from build123d import *

# Parameters (mm, degrees)
SKETCH1_R                    = 33.274
BOSS_EXTRUDE1_DEPTH          = 6.35
PLATEMTGSCREW_D              = 2.8702
PLATEMTGSCREW_DEPTH          = 10.1854
PLATEMTGSCREW_CSINK_D        = 7.7978
PLATEMTGSCREW_CSINK_ANGLE    = 82
PLATEMTGSCREW_TIP            = 0.862295074
ENCODERMTGHOLES_D            = 2.2606
SLIPRGSHFTCLR_D              = 13.09624
SLIPRGSHFTCLR_DEPTH          = 6.35
SLIPRGSHFTCLR_TIP            = 3.934507437
ADDITIONAL_HOLES_D           = 4.0386
ADDITIONAL_HOLES_CSINK_D     = 7.7978
ADDITIONAL_HOLES_CSINK_ANGLE = 82
CUT_EXTRUDE1_DEPTH           = 7.3500001


with BuildPart() as part:
    # Sketch1 → Boss-Extrude1 (new body)
    with BuildSketch(Plane(origin=(0, 0, 0), x_dir=(1, 0, 0), z_dir=(0, 1, 0))):
        Circle(SKETCH1_R)
    extrude(amount=BOSS_EXTRUDE1_DEPTH)

    # PlateMtgScrew
    with Locations(Plane(origin=(0, 6.35, 0), x_dir=(1, 0, 0), z_dir=(0, 1, 0))):
        with Locations((30.226, 0), (-30.226, 0), (0, -30.226)):
            CounterSinkHole(PLATEMTGSCREW_D / 2, PLATEMTGSCREW_CSINK_D / 2, depth=PLATEMTGSCREW_DEPTH, counter_sink_angle=PLATEMTGSCREW_CSINK_ANGLE)
            with Locations((0, 0, -(PLATEMTGSCREW_DEPTH + PLATEMTGSCREW_TIP / 2))):  # 118° drill point
                Cone(0, PLATEMTGSCREW_D / 2, PLATEMTGSCREW_TIP, mode=Mode.SUBTRACT)

    # EncoderMtgHoles (through all)
    with Locations(Plane(origin=(0, 6.35, 0), x_dir=(1, 0, 0), z_dir=(0, 1, 0))):
        with Locations((23.0124, 0), (-23.0124, 0)):
            Hole(ENCODERMTGHOLES_D / 2)

    # SlipRgShftClr
    with Locations(Plane(origin=(0, 6.35, 0), x_dir=(1, 0, 0), z_dir=(0, 1, 0))):
        with Locations((0, 0)):
            Hole(SLIPRGSHFTCLR_D / 2, depth=SLIPRGSHFTCLR_DEPTH)
            with Locations((0, 0, -(SLIPRGSHFTCLR_DEPTH + SLIPRGSHFTCLR_TIP / 2))):  # 118° drill point
                Cone(0, SLIPRGSHFTCLR_D / 2, SLIPRGSHFTCLR_TIP, mode=Mode.SUBTRACT)

    # Additional Holes (through all)
    with Locations(Plane(origin=(0, 6.35, 0), x_dir=(1, 0, 0), z_dir=(0, 1, 0))):
        with Locations((-9.898670365, 5.715), (9.898670365, 5.715)):
            CounterSinkHole(ADDITIONAL_HOLES_D / 2, ADDITIONAL_HOLES_CSINK_D / 2, counter_sink_angle=ADDITIONAL_HOLES_CSINK_ANGLE)

    # Sketch16 → Cut-Extrude1 (cut, through all)
    with BuildSketch(Plane(origin=(0, 6.35, 0), x_dir=(1, 0, 0), z_dir=(0, 1, 0))):
        Polygon((-192.02067324, 25.4), (-21.494163766, 25.4), (21.494163766, 25.4), (192.02067324, 25.4), (192.02067324, 366.453018948), (-192.02067324, 366.453018948), align=None)
    extrude(amount=-CUT_EXTRUDE1_DEPTH, mode=Mode.SUBTRACT)


solid = part.part
Design review of the part built by this model. Coordinates are the model's own, in mm. Give positions to 0.01 mm unless a question says otherwise; leave off trailing zeros. Loops run counter-clockwise (first coordinate to the right, second up) from the corner with the lowest first, then second, coordinate; pieces in that order, holes last. Notation, with made-up numbers: M 62.5,78.5 L 107.5,78.5 A16 cw 107.5,92.5 Z; hole C 3.5,15.25 d2. An arc over 180 degrees is marked long. One line per question, with ' | ' between items. Start each with the question number.
1. Add section A-A (z = 0). Write out the cut boundary in (x, y), plus the area to 3 significant figures.
2. To check wall thickness, follow L1, parallel to Z at x = 0, y = 3; L2, parallel to Z at x = -2, y = 5.75; L3, parallel to X at y = 2.75, z = -7. State the ranges of each line that lie inside material, in increasing order.
3. Insertion check: P1, Ø1.7, axis at x = 0, z = 30.226, coming from the +Y side; P2, Ø3, axis at x = 20, y = 5, coming from the +Z side; P3, Ø4.5, axis at x = -30.226, z = 0, coming from the +Y side. Each pin has a flat end and moves straight along its axis. Give the tip position at first contact, or say it passes through.
4. Add section C-C (y = 1.5). Give the number of separate pieces and of enclosed holes in the cut face, plus the area to 3 significant figures.
5. Add section B-B (x = 0). Write out the cut boundary in (y, z), plus the area to 3 significant figures.
6. Add section D-D (z = 24). Write out the cut boundary in (x, y), plus the area to 3 significant figures.
7. The part is to be moulded in two halves that separate along X. For faces 1 (the face through (-1.136, 3.131, 33.255)), 2 (the face through (0.311, 1.733, 31.627)), 3 (the face through (7, 6.35, 3)), 4 (the face through (0.202, 3.653, 28.684)), say which applies: released by +X, released by -X, zero draft, split by the parting line, or undercut.
Worked out:
1) outline: M -33.27,0 L -31.66,0 L -31.66,3.52 L -33.27,5.37 Z; M -28.79,0 L -24.14,0 L -24.14,6.35 L -26.33,6.35 L -28.79,3.52 Z; M -21.88,0 L -6.55,0 L -6.55,6.35 L -21.88,6.35 Z; M 6.55,0 L 21.88,0 L 21.88,6.35 L 6.55,6.35 Z; M 24.14,0 L 28.79,0 L 28.79,3.52 L 26.33,6.35 L 24.14,6.35 Z; M 31.66,0 L 33.27,0 L 33.27,5.37 L 31.66,3.52 Z | area: 261 mm²
2) L1: z = -25.4 to -6.55, 6.55 to 28.79, 31.66 to 33.27 | L2: z = -25.4 to -6.24, 6.24 to 27.5, 32.95 to 33.21 | L3: x = -32.53 to -11.46, -8.34 to 8.34, 11.46 to 32.53
3) P1: passes through | P2: stops at z = 27.66 | P3: stops at y = 4.45
4) separate pieces: 1 | enclosed holes: 8 | area: 3,060 mm²
5) outline: M 0,-25.4 L 6.35,-25.4 L 6.35,-6.55 L 0,-6.55 Z; M 0,6.55 L 6.35,6.55 L 6.35,26.33 L 3.52,28.79 L 0,28.79 Z; M 0,31.66 L 3.52,31.66 L 5.37,33.27 L 0,33.27 Z | area: 265 mm²
6) outline: M -23.05,0 L 23.05,0 L 23.05,6.35 L -23.05,6.35 Z | area: 293 mm²
7) face 1: split by the parting line | face 2: undercut | face 3: zero draft | face 4: undercut
